Model file for the job. Use its own axes, mm. Coordinates: 2 decimals unless noted, no trailing zeros. Order: outer loops, then holes, each group sorted by start corner. A loop starts at its lowest first (then second) coordinate and runs counter-clockwise, first axis right, second up. Notation, with made-up numbers: M -1,-10 L 24,-10 A19 ccw 24,11 Z; hole C 40,7.25 d9. An arc over 180 degrees is marked long. Return JSON: item names as keys, results as strings.
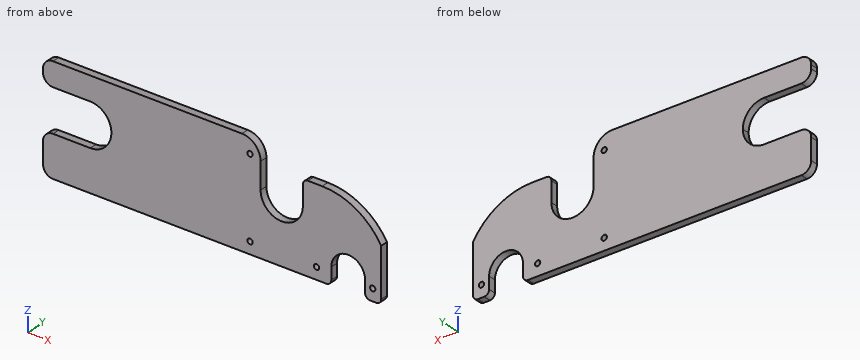
```python
from build123d import *

# Parameters (mm, degrees)
BOSS_EXTRUDE2_DEPTH     = 9.525
CUT_EXTRUDE2_DEPTH      = 10.525
F_1_4_CLEARANCE_HOLE1_D = 6.7564
FILLET5_R               = 23.8125
FILLET6_R               = 12.7
FILLET7_R               = 6.35


with BuildPart() as part:
    # Sketch1 → Boss-Extrude2 (new body)
    with BuildSketch(Plane(origin=(0, 0, 0), x_dir=(1, 0, 0), z_dir=(0, 1, 0))):
        with BuildLine():
            Line((25.4, 0), (277.8125, 0))
            Line((277.8125, 0), (277.8125, 57.15))
            ThreePointArc((277.8125, 57.15), (304.8, 84.1375), (331.78749993, 57.15))
            Line((331.78749993, 57.15), (331.78749993, 0))
            Line((331.78749993, 0), (357.18749993, 0))
            ThreePointArc((357.18749993, 0), (407.751306336, 19.640432558), (431.8, 68.2625))
            Line((431.8, 68.2625), (431.8, 136.525))
            Line((431.8, 136.525), (411.226, 136.525))
            Line((411.226, 136.525), (411.226, 114.935))
            ThreePointArc((411.226, 114.935), (389.636, 93.345), (368.046, 114.935))
            Line((368.046, 114.935), (368.046, 136.525))
            Line((368.046, 136.525), (23.8125, 136.525))
            Line((23.8125, 136.525), (12.7, 136.525))
            ThreePointArc((12.7, 136.525), (3.719743879, 132.805256121), (0, 123.825))
            Line((0, 123.825), (0, 96.8375))
            Line((0, 96.8375), (0, 84.1375))
            Line((0, 84.1375), (22.225, 84.1375))
            Line((22.225, 84.1375), (60.325, 84.1375))
            ThreePointArc((60.325, 84.1375), (79.408044257, 76.233044257), (87.3125, 57.15))
            ThreePointArc((87.3125, 57.15), (79.408044257, 38.066955743), (60.325, 30.1625))
            Line((60.325, 30.1625), (22.225, 30.1625))
            Line((22.225, 30.1625), (0, 30.1625))
            Line((0, 30.1625), (0, 17.4625))
            Line((0, 17.4625), (0, 12.7))
            ThreePointArc((0, 12.7), (3.719743879, 3.719743879), (12.7, 0))
            Line((12.7, 0), (25.4, 0))
        make_face()
    extrude(amount=BOSS_EXTRUDE2_DEPTH)

    # Sketch2 → Cut-Extrude2 (cut, through all)
    with BuildSketch(Plane(origin=(0, 9.525, 0), x_dir=(1, 0, 0), z_dir=(0, 1, 0))):
        with BuildLine():
            Line((331.78749993, 0), (331.78749993, 25.4))
            Line((331.78749993, 25.4), (356.39375, 25.4))
            ThreePointArc((356.39375, 25.4), (399.762219091, 36.86444095), (431.8, 68.2625))
            ThreePointArc((431.8, 68.2625), (407.751306336, 19.640432558), (357.18749993, 0))
            Line((357.18749993, 0), (331.78749993, 0))
        make_face()
    extrude(amount=-CUT_EXTRUDE2_DEPTH, mode=Mode.SUBTRACT)

    # 1/4 Clearance Hole1 (through all)
    with Locations(Plane(origin=(0, 9.525, 0), x_dir=(1, 0, 0), z_dir=(0, 1, 0))):
        with Locations((420.9542, 121.44375), (349.26905, 121.44375), (264.318750035, 121.44375), (264.318750035, 19.84375)):
            Hole(F_1_4_CLEARANCE_HOLE1_D / 2)

    # Fillet5
    fillet5_edges = [part.edges().sort_by_distance(p)[0] for p in [
        (277.8125, 4.7625, 0),
    ]]
    fillet(fillet5_edges, radius=FILLET5_R)

    # Fillet6
    fillet6_edges = [part.edges().sort_by_distance(p)[0] for p in [
        (0, 4.7625, -84.1375),
        (0, 4.7625, -30.1625),
    ]]
    fillet(fillet6_edges, radius=FILLET6_R)

    # Fillet7
    fillet7_edges = [part.edges().sort_by_distance(p)[0] for p in [
        (431.8, 4.7625, -136.525),
        (411.226, 4.7625, -136.525),
        (368.046, 4.7625, -136.525),
        (331.78749993, 4.7625, -25.4),
    ]]
    fillet(fillet7_edges, radius=FILLET7_R)


solid = part.part
```
Item 1: Saw through at A-A (z = -42.5). Write the cut outline in (x, y) (1 decimal), and give its area (3 significant figures).
Check result:
{"outline": "M 83,0 L 277.8,0 L 277.8,9.5 L 83,9.5 Z; M 331.8,0 L 408.4,0 L 408.4,9.5 L 331.8,9.5 Z", "area": "2,590 mm2"}
Item 2: Wall check: line 1 (X direction, y = 5.75, z = -122); line 2 (X direction, y = 6, z = -123); line 3 (Z direction, x = 57, y = 4) (1 decimal). Give the ranges that are in metal, low to high.
Check result:
{"line 1": "x = 0 to 260.99, 267.65 to 345.94, 352.6 to 368.05, 411.23 to 417.62, 424.29 to 431.8", "line 2": "x = 0 to 261.32, 267.32 to 346.27, 352.27 to 368.05, 411.23 to 417.96, 423.95 to 431.8", "line 3": "z = -136.5 to -84.1, -30.2 to 0"}
Item 3: Saw through at C-C (x = 78). Write the cut outline in (y, z) (3 decimals).
Check result:
{"outline": "M 0,-136.525 L 9.525,-136.525 L 9.525,-77.544 L 0,-77.544 Z; M 0,-36.756 L 9.525,-36.756 L 9.525,0 L 0,0 Z"}
Item 4: Saw through at D-D (x = 304.8). Write the cut outline in (y, z) (1 decimal).
Check result:
{"outline": "M 0,-136.5 L 9.5,-136.5 L 9.5,-84.1 L 0,-84.1 Z"}
Item 5: Saw through at B-B (y = 4.5). Count the separate pieces of the cut face and the enclosed holes in it, and give its area (3 significant figures).
Check result:
{"separate pieces": "1", "enclosed holes": "4", "area": "44,700 mm2"}
Item 6: Drop flat-ended pins along their axis: pin 1 Ø4 at (x, z) = (358, -105.5) entering from -Y; pin 2 Ø3 at (x, y) = (345.5, 7) entering from +Z. Give the stop position or say it passes through.
Check result:
{"pin 1": "stops at y = 0", "pin 2": "stops at z = -25.4"}
